```python
from build123d import *

# Parameters (mm, degrees)
BOSS_EXTRUDE1_DEPTH = 31.75
SKETCH2_R           = 19.05
SKETCH2_R_2         = 15.875
BOSS_EXTRUDE2_DEPTH = 762


with BuildPart() as part:
    # Sketch1 → Boss-Extrude1 (new body, symmetric)
    with BuildSketch(Plane(origin=(0, 0, 0), x_dir=(1, 0, 0), z_dir=(0, 1, 0))):
        Polygon((0, 31.75), (0, -31.75), (-76.2, -31.75), (-76.2, -25.4), (-6.35, -25.4), (-6.35, 31.75), align=None)
    extrude(amount=BOSS_EXTRUDE1_DEPTH, both=True)

    # Sketch2 → Boss-Extrude2 (add)
    with BuildSketch(Plane.XY.offset(31.75)):
        with Locations((-50.8, 0)):
            Circle(SKETCH2_R)
        with Locations((-50.8, 0)):
            Circle(SKETCH2_R_2, mode=Mode.SUBTRACT)
    extrude(amount=BOSS_EXTRUDE2_DEPTH)


solid = part.part
```
Design review of the part built by this model. Coordinates are the model's own, in mm. A direction names the side the tool comes from. Give positions to 0.01 mm unless a question says otherwise; leave off trailing zeros. Write each loop counter-clockwise with the first axis right and the second up, starting at its lowest first coordinate (ties: lowest second). Pieces come first, ordered by that corner, then holes. Notation, with made-up numbers: (65, 85.5) -> (116, 85.5) arc R15 cw to (116, 100.5) -> close; hole circle Ø4 at (0.25, -33). An arc over 180 degrees is marked (long way). Answer in a Markdown table with one row per item.
(1) To check wall thickness, follow probe 1 along Y at (x, z) = (-50.8, 331.5) (3 decimals); probe 2 along X at (y, z) = (-2, 523); probe 3 along Z at (x, y) = (-32, -16.5). State the ranges of each line that lie inside material, in increasing order.
Results:
| item | result |
|---|---|
| probe 1 | -19.05 to -15.875, 15.875 to 19.05 |
| probe 2 | -69.74 to -66.55, -35.05 to -31.86 |
| probe 3 | 25.4 to 31.75 |
(2) Mouldability with a two-part tool opening along Y and no side actions: class faces 4 (the cylindrical face through (-33.203, -7.296, 407.416)), 5 (the cylindrical face through (-36.136, -6.08, 407.416)), 6 (the flat face through (-24, -31.75, 26)), 7 (the flat face through (-6.35, 0, -3)) as +Y half, -Y half, draft (parallel to the pull), parting line (faces both ways), or undercut.
Results:
| item | result |
|---|---|
| face 4 | parting line |
| face 5 | undercut |
| face 6 | -Y half |
| face 7 | draft |
(3) Consider section C-C (z = 613.5). State the section outline as (x, y) points (3 decimals), then the cut area to 3 significant figures.
Results:
| item | result |
|---|---|
| outline | circle Ø38.1 at (-50.8, 0); hole circle Ø31.75 at (-50.8, 0) |
| area | 348 mm2 |
(4) For faces 1 (the flat face through (-51, 0, 31.75)), 2 (the flat face through (-42, 0, 25.4)), 3 (the flat face through (0, 0, 0)), list the 3-axis set-ups (+Z, -Z, +X, -X, +Y, -Y) from which the entire face can be reached by the end or side of a thin tool; tool diameter is ignored.
Results:
| item | result |
|---|---|
| face 1 | +Z |
| face 2 | -Z, -X, +Y, -Y |
| face 3 | +Z, -Z, +X, +Y, -Y |
(5) Consider section A-A (x = -50.8). State the section outline as (y, z) points (3 decimals).
Results:
| item | result |
|---|---|
| outline | (-31.75, 25.4) -> (31.75, 25.4) -> (31.75, 31.75) -> (19.05, 31.75) -> (19.05, 793.75) -> (15.875, 793.75) -> (15.875, 31.75) -> (-15.875, 31.75) -> (-15.875, 793.75) -> (-19.05, 793.75) -> (-19.05, 31.75) -> (-31.75, 31.75) -> close |
(6) Consider section B-B (y = 0). State the section outline as (x, z) points (3 decimals).
Results:
| item | result |
|---|---|
| outline | (-76.2, 25.4) -> (-6.35, 25.4) -> (-6.35, -31.75) -> (0, -31.75) -> (0, 31.75) -> (-31.75, 31.75) -> (-31.75, 793.75) -> (-34.925, 793.75) -> (-34.925, 31.75) -> (-66.675, 31.75) -> (-66.675, 793.75) -> (-69.85, 793.75) -> (-69.85, 31.75) -> (-76.2, 31.75) -> close |
(7) Clearance check with flat-ended pins moving along their axes: pin 1 (12 mm diameter, centred on x = -47.5, y = -8, fed in from +Z); pin 2 (6 mm diameter, centred on y = -10.5, z = 515, fed in from -X); pin 3 (6 mm diameter, centred on y = 18.5, z = 603, fed in from +X). State where each tip first meets the part, or that it passes through.
Results:
| item | result |
|---|---|
| pin 1 | z = 31.75 |
| pin 2 | x = -68.31 |
| pin 3 | x = -39.73 |
